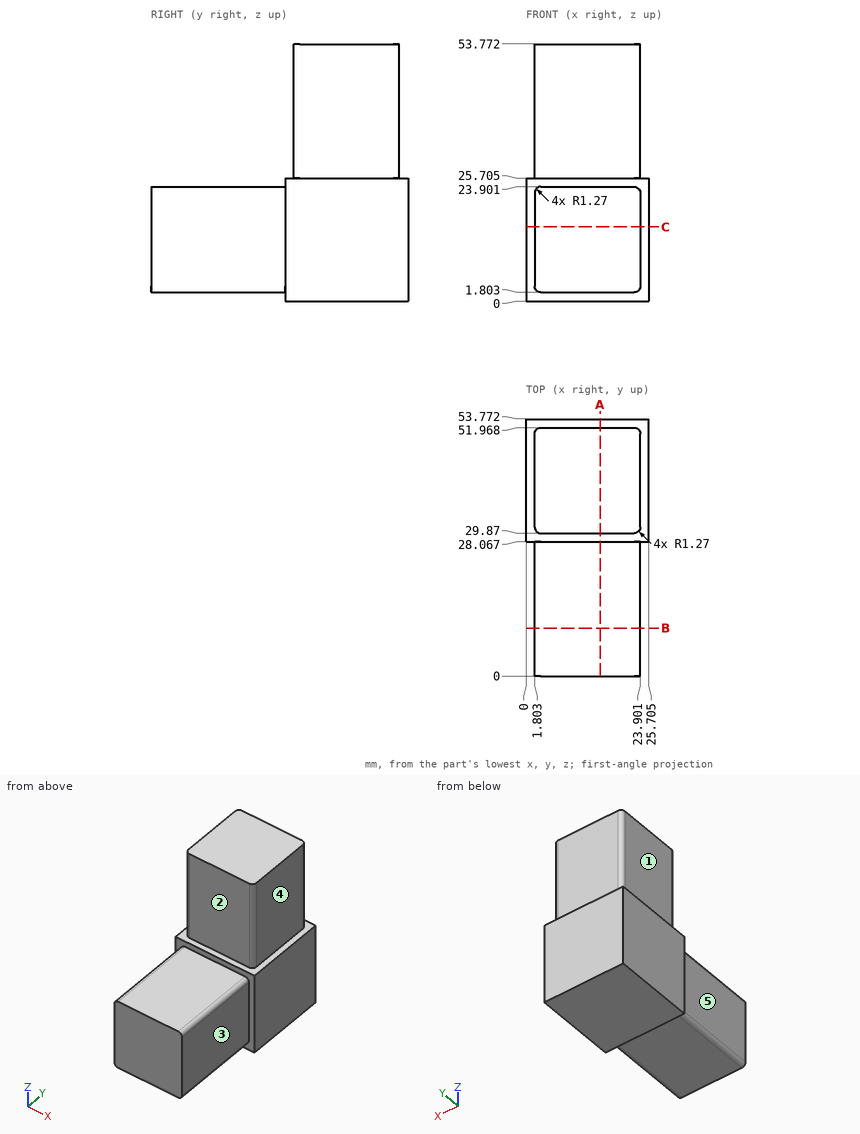
Could you check a few things on this drawing? It's one solid part, dimensions in mm from its lowest x, y, z. A direction names the side the tool comes from. Coordinates: 2 decimals unless noted, no trailing zeros. Order: outer loops, then holes, each group sorted by start corner. A loop starts at its lowest first (then second) coordinate and runs counter-clockwise, first axis right, second up.
1) Imagine slicing it at B-B on y = 10. List the corners of the cut face in (x, z) for me, and give its area (3 significant figures).
2) Imagine slicing it at C-C on z = 15.5. List the corners of the cut face in (x, y) for me (1 decimal), and give its area (3 significant figures).
3) Which directions (+Z, -Z, +X, -X, +Y, -Y) give clear straight access to the entire face, cutting with the end or side of a thin tool? Please do the marked faces 1, 2, 3, 4 and 5.
4) Imagine slicing it at A-A on x = 15.5. List the corners of the cut face in (y, z) for me (1 decimal), and give its area (3 significant figures).
5) I need wall thicknesses on line 1 (X direction, y = 10, z = 14); line 2 (Y direction, x = 4.25, z = 37.5). Which ranges of each line are inside material? Lowest first, please.
6) Will these pins go through, and if not, where does the flat tip stop? pin 1 (15.5 mm diameter, centred on y = 9.5, z = 11, fed in from +X); pin 2 (12 mm diameter, centred on y = 22.5, z = 31, fed in from -X); pin 3 (6 mm diameter, centred on y = 9, z = 9, fed in from -X); pin 4 (2 mm diameter, centred on x = 6, y = 17, fed in from +Z).
Response values:
1. outline: (1.8, 3.07) arc R1.27 ccw to (3.07, 1.8) - (22.63, 1.8) arc R1.27 ccw to (23.9, 3.07) - (23.9, 22.63) arc R1.27 ccw to (22.63, 23.9) - (3.07, 23.9) arc R1.27 ccw to (1.8, 22.63) - close
1. area: 487 mm2
2. outline: (0, 28.1) - (1.8, 28.1) - (1.8, 0) - (23.9, 0) - (23.9, 28.1) - (25.7, 28.1) - (25.7, 53.8) - (0, 53.8) - close
2. area: 1,280 mm2
3. face 1: +Z, -X, +Y, -Y
3. face 2: +Z, +X, -X, -Y
3. face 3: +Z, -Z, +X, -Y
3. face 4: +Z, +X, +Y, -Y
3. face 5: +Z, -Z, -X, -Y
4. outline: (0, 1.8) - (28.1, 1.8) - (28.1, 0) - (53.8, 0) - (53.8, 25.7) - (52, 25.7) - (52, 53.8) - (29.9, 53.8) - (29.9, 25.7) - (28.1, 25.7) - (28.1, 23.9) - (0, 23.9) - close
4. area: 1,900 mm2
5. line 1: x = 1.8 to 23.9
5. line 2: y = 29.87 to 51.97
6. pin 1: stops at x = 23.9
6. pin 2: passes through
6. pin 3: stops at x = 1.8
6. pin 4: stops at z = 23.9
